from build123d import *

# Parameters (mm, degrees)
SKETCH1_R           = 1.5
SKETCH1_W           = 5
SKETCH1_H           = 5
BOSS_EXTRUDE1_DEPTH = 5
FILLET1_R           = 4


with BuildPart() as part:
    # Sketch1 → Boss-Extrude1 (new body)
    with BuildSketch(Plane.XY):
        with BuildLine():
            Line((-21, 80), (-31, 80))
            ThreePointArc((-31, 80), (-29.085023859, 69.273332897), (-23.576684701, 59.871911702))
            Line((-23.576684701, 59.871911702), (-23.576684701, 0))
            Line((-23.576684701, 0), (-36.012504096, -70.527036447))
            Line((-36.012504096, -70.527036447), (-16.316349035, -74))
            Line((-16.316349035, -74), (-7.5, -24))
            Line((-7.5, -24), (7.5, -24))
            Line((7.5, -24), (16.316349035, -74))
            Line((16.316349035, -74), (36.012504096, -70.527036447))
            Line((36.012504096, -70.527036447), (23.576684701, 0))
            Line((23.576684701, 0), (23.576684701, 59.871911702))
            ThreePointArc((23.576684701, 59.871911702), (29.085023859, 69.273332897), (31, 80))
            Line((31, 80), (21, 80))
            ThreePointArc((21, 80), (0, 59), (-21, 80))
        make_face()
        Circle(SKETCH1_R, mode=Mode.SUBTRACT)
        with Locations((0, 45)):
            Circle(SKETCH1_R, mode=Mode.SUBTRACT)
        with Locations((-7.5, 0)):
            Rectangle(SKETCH1_W, SKETCH1_H, mode=Mode.SUBTRACT)
        with Locations((7.5, 0)):
            Rectangle(SKETCH1_W, SKETCH1_H, mode=Mode.SUBTRACT)
        with Locations((-7.5, 45)):
            Rectangle(SKETCH1_W, SKETCH1_H, mode=Mode.SUBTRACT)
        with Locations((7.5, 45)):
            Rectangle(SKETCH1_W, SKETCH1_H, mode=Mode.SUBTRACT)
    extrude(amount=BOSS_EXTRUDE1_DEPTH)

    # Fillet1
    fillet1_edges = [part.edges().sort_by_distance(p)[0] for p in [
        (21, 80, 2.5),
        (31, 80, 2.5),
        (23.576684701, 59.871911702, 2.5),
        (23.576684701, 0, 2.5),
        (36.012504096, -70.527036447, 2.5),
        (16.316349035, -74, 2.5),
        (7.5, -24, 2.5),
        (-7.5, -24, 2.5),
        (-16.316349035, -74, 2.5),
        (-36.012504096, -70.527036447, 2.5),
        (-23.576684701, 0, 2.5),
        (-23.576684701, 59.871911702, 2.5),
        (-31, 80, 2.5),
        (-21, 80, 2.5),
    ]]
    fillet(fillet1_edges, radius=FILLET1_R)


solid = part.part
Verification items for the finished model (mm, model axes). A direction names the side the tool comes from. Coordinates: 2 decimals unless noted, no trailing zeros. Order: outer loops, then holes, each group sorted by start corner. A loop starts at its lowest first (then second) coordinate and runs counter-clockwise, first axis right, second up. Notation, with made-up numbers: M 80,27 L 115,27 A32 cw 115,66 Z; hole C 26.25,18.25 d9. An arc over 180 degrees is marked long. One line per item, written item: value. Start each with the question number.
Item 1: Depth check by flat-ended pin: P1, Ø2.5, axis at y = -0.5, z = 2, coming from the +X side; P2, Ø1.5, axis at y = -1, z = 1.5, coming from the -X side; P3, Ø3, axis at x = 10.5, z = 3.5, coming from the +Y side. Enter the tip coordinate at first touch or a pass-through.
Item 2: Access from +Z, -Z, +X, -X, +Y, -Y to the whole of each face (thin tool, end or side, straight path). Record for faces 1 (the flat face through (23.577, 29, 2)), 2 (the cylindrical face through (-22.116, 79.072, 2.535)), 3 (the flat face through (0, -24, 2)), 4 (the flat face through (-8, 42.5, 2)).
Item 3: Sectioned sample at D-D on y = -10. Record the cut outline in (x, z), then the cut area to 3 significant figures.
Item 4: Sectioned sample at B-B on x = 0. Record the cut outline in (y, z), then the cut area to 3 significant figures.
Item 5: Thickness scan on probe 1 along Y at (x, z) = (0, 3.95); probe 2 along Y at (x, z) = (-7.5, 1.8); probe 3 along X at (y, z) = (32, 2.1). Record the ranges inside material, lowest first.
Item 6: Mould release check, pull along Y, two halves, no side actions. Record for faces 5 (the flat face through (0, 4, 0)), 6 (the cylindrical face through (6.685, -24.911, 2.535)), 7 (the flat face through (10, 0, 2)): pulls with the +Y half, pulls with the -Y half, needs draft (parallel to the pull), parting line crosses it, or undercut.
Item 7: Sectioned sample at C-C on z = 2. Give the number of separate pieces and of enclosed holes in the cut face, then the cut area to 3 significant figures.
Item 8: Sectioned sample at A-A on y = 45. Record the cut outline in (x, z).
Calculated:
1. P1: x = 23.89
1. P2: x = -23.89
1. P3: y = 62.77
2. face 1: +Z, -Z, +X
2. face 2: +Z, -Z, +Y
2. face 3: +Z, -Z, -Y
2. face 4: +Z, -Z
3. outline: M -25.34,0 L 25.34,0 L 25.34,5 L -25.34,5 Z
3. area: 253 mm^2
4. outline: M -24,0 L -1.5,0 L -1.5,5 L -24,5 Z; M 1.5,0 L 43.5,0 L 43.5,5 L 1.5,5 Z; M 46.5,0 L 59,0 L 59,5 L 46.5,5 Z
4. area: 385 mm^2
5. probe 1: -24 to -1.5, 1.5 to 43.5, 46.5 to 59
5. probe 2: -25.82 to -2.5, 2.5 to 42.5, 47.5 to 60.38
5. probe 3: -23.58 to 23.58
6. face 5: needs draft
6. face 6: pulls with the -Y half
6. face 7: undercut
7. separate pieces: 1
7. enclosed holes: 6
7. area: 6,340 mm^2
8. outline: M -23.58,0 L -10,0 L -10,5 L -23.58,5 Z; M -5,0 L -1.5,0 L -1.5,5 L -5,5 Z; M 1.5,0 L 5,0 L 5,5 L 1.5,5 Z; M 10,0 L 23.58,0 L 23.58,5 L 10,5 Z
